Can you work these out from the model? Positions are in its coordinate system, mm. Coordinates: 2 decimals unless noted, no trailing zeros. Order: outer loops, then holes, each group sorted by start corner. A loop starts at its lowest first (then second) coordinate and runs counter-clockwise, first axis right, second up. Notation, with made-up numbers: (53, -25) -> (101, -25) arc R28 cw to (101, 9) -> close; hole circle Ø5 at (79, -18). An arc over 180 degrees is marked (long way). Answer in a Markdown table with one row per item.
```python
from build123d import *

# Parameters (mm, degrees)
F0_W     = 40
F0_H     = 40
F1_DEPTH = 5
F2_R     = 10.3
F3_DEPTH = 5.001
F6_D     = 3
F7_D     = 4
F8_R     = 5


with BuildPart() as f1:
    # F0 (on Top) → F1 (new body)
    with BuildSketch(Plane.XY):
        Rectangle(F0_W, F0_H)
    extrude(amount=F1_DEPTH)

    # F2 (on face) → F3 (cut, through all)
    with BuildSketch(Plane.XY.offset(5)):
        Circle(F2_R)
    extrude(amount=-F3_DEPTH, mode=Mode.SUBTRACT)

    # F6 (through all)
    with Locations(Plane.XY.offset(5)):
        with Locations((-15.5, 15.5), (15.5, 15.5), (15.5, -15.5), (-15.5, -15.5)):
            Hole(F6_D / 2)

    # F7 (through all)
    with Locations(Plane.XY.offset(5)):
        with Locations((-15, 0), (15, 0)):
            Hole(F7_D / 2)

    # F8
    f8_edges = [f1.edges().sort_by_distance(p)[0] for p in [
        (-20, 20, 2.5),
        (20, 20, 2.5),
        (-20, -20, 2.5),
        (20, -20, 2.5),
    ]]
    fillet(f8_edges, radius=F8_R)


solid = f1.part
```
(1) Suppose I cut it at B-B (z = 3.6). Please give me the cut outline in (x, y).
Response values:
| item | result |
|---|---|
| outline | (-20, -15) arc R5 ccw to (-15, -20) -> (15, -20) arc R5 ccw to (20, -15) -> (20, 15) arc R5 ccw to (15, 20) -> (-15, 20) arc R5 ccw to (-20, 15) -> close; hole circle Ø3 at (-15.5, -15.5); hole circle Ø4 at (-15, 0); hole circle Ø3 at (-15.5, 15.5); hole circle Ø20.6 at (0, 0); hole circle Ø4 at (15, 0); hole circle Ø3 at (15.5, -15.5); hole circle Ø3 at (15.5, 15.5) |
(2) Will this pin go through, and if not, where does the flat tip stop? pin 1 Ø3 at (x, y) = (15, 0) entering from -Z.
Response values:
| item | result |
|---|---|
| pin 1 | through |
(3) I need wall thicknesses on line 1 (Y direction, x = 15, z = 2.7); line 2 (Y direction, x = 0, z = 2.6); line 3 (Y direction, x = 15.5, z = 2.75). Which ranges of each line are inside material? Lowest first, please. Write a range as [from, to].
Response values:
| item | result |
|---|---|
| line 1 | [-20, -16.91], [-14.09, -2], [2, 14.09], [16.91, 20] |
| line 2 | [-20, -10.3], [10.3, 20] |
| line 3 | [-19.97, -17], [-14, -1.94], [1.94, 14], [17, 19.97] |
(4) Suppose I cut it at D-D (y = -9). Please give me the cut outline in (x, z), and give its area (3 significant figures).
Response values:
| item | result |
|---|---|
| outline | (-20, 0) -> (-5.01, 0) -> (-5.01, 5) -> (-20, 5) -> close; (5.01, 0) -> (20, 0) -> (20, 5) -> (5.01, 5) -> close |
| area | 150 mm2 |
(5) We'd pull the mould along X, two halves only. Please class faces 1 (the cylindrical face through (-13.4, -1.2, 2.5)), 2 (the flat face through (-20, 0, 2)), 3 (the flat face through (-9, 9, 0)): +X half, -X half, draft (parallel to the pull), parting line (faces both ways), or undercut.
Response values:
| item | result |
|---|---|
| face 1 | undercut |
| face 2 | -X half |
| face 3 | draft |
(6) Suppose I cut it at C-C (y = 0). Please give me the cut outline in (x, z).
Response values:
| item | result |
|---|---|
| outline | (-20, 0) -> (-17, 0) -> (-17, 5) -> (-20, 5) -> close; (-13, 0) -> (-10.3, 0) -> (-10.3, 5) -> (-13, 5) -> close; (10.3, 0) -> (13, 0) -> (13, 5) -> (10.3, 5) -> close; (17, 0) -> (20, 0) -> (20, 5) -> (17, 5) -> close |
(7) Suppose I cut it at A-A (x = 0). Please give me the cut outline in (y, z), and give its area (3 significant figures).
Response values:
| item | result |
|---|---|
| outline | (-20, 0) -> (-10.3, 0) -> (-10.3, 5) -> (-20, 5) -> close; (10.3, 0) -> (20, 0) -> (20, 5) -> (10.3, 5) -> close |
| area | 97.0 mm2 |
